Print and shaded views of the part. All mm, measured from the part's lowest x, y and z. A direction names the side the tool comes from. Round coordinates to 2 decimals unless told otherwise and drop trailing zeros. Loops run counter-clockwise (first coordinate to the right, second up) from the corner with the lowest first, then second, coordinate; pieces in that order, holes last. Notation, with made-up numbers: (60, 76.25) -> (84, 76.25) arc R34 cw to (84, 115.25) -> close; hole circle Ø2 at (38.25, 64). An arc over 180 degrees is marked (long way). Use a Markdown table: item, result.
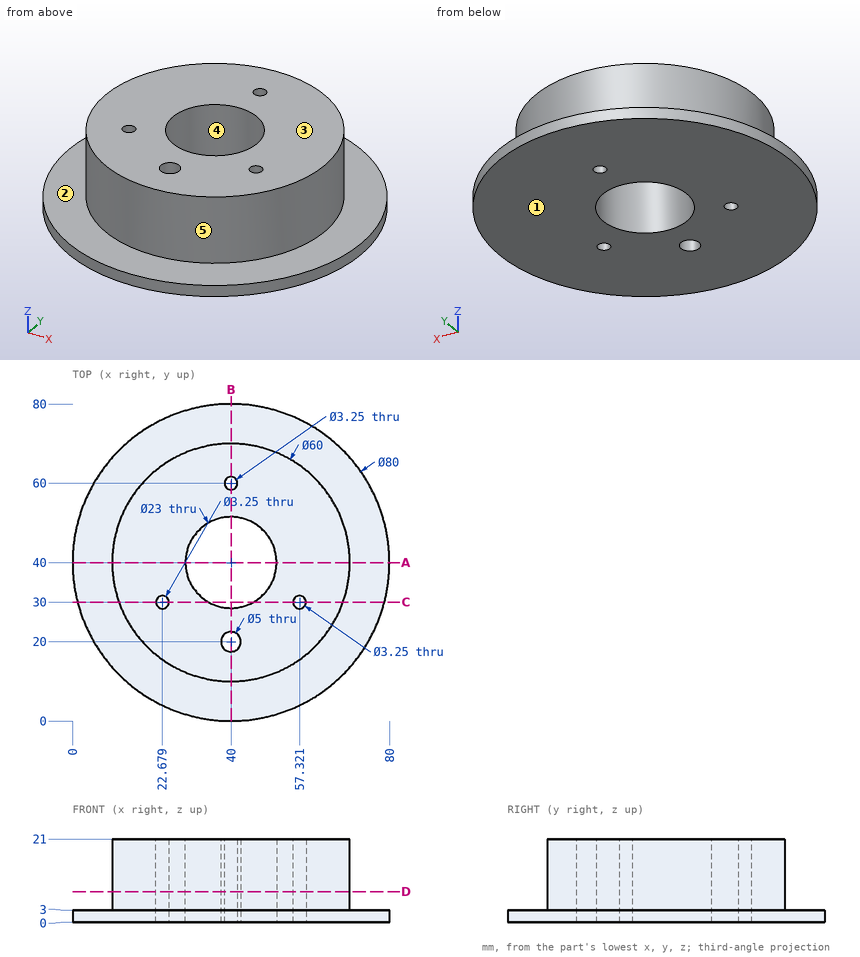
Q1. Tool access for the marked faces 1 and 2: list every direction of +Z, -Z, +X, -X, +Y, -Y with a clear straight run to the whole face (end or side of a thin tool).
Results list:
| item | result |
|---|---|
| face 1 | -Z, +X, -X, +Y, -Y |
| face 2 | +Z |
Q2. Band-saw the part on A-A, the plane y = 40. Give the cut face in (x, z), plus the area to 3 significant figures.
Results list:
| item | result |
|---|---|
| outline | (0, 0) -> (28.5, 0) -> (28.5, 21) -> (10, 21) -> (10, 3) -> (0, 3) -> close; (51.5, 0) -> (80, 0) -> (80, 3) -> (70, 3) -> (70, 21) -> (51.5, 21) -> close |
| area | 837 mm² |
Q3. Drill centre lines: L1, parallel to Y at x = 40, z = 12.25 (1 decimal); L2, parallel to Z at x = 55, y = 6; L3, parallel to X at y = 46, z = 13.75 (1 decimal). Where is each one in solid material? Low to high. Write a range as from..to.
Results list:
| item | result |
|---|---|
| L1 | y = 10..17.5, 22.5..28.5, 51.5..58.4, 61.6..70 |
| L2 | z = 0..3 |
| L3 | x = 10.6..30.2, 49.8..69.4 |
Q4. Flat gauge pins, fed straight in: pin 1 (6 mm diameter, centred on x = 40, y = 20, fed in from +Z); pin 2 (4 mm diameter, centred on x = 17, z = 17.5, fed in from -Y) (1 decimal); pin 3 (6 mm diameter, centred on y = 55.5, z = 4, fed in from -X); pin 4 (2 mm diameter, centred on y = 29.5, z = 3, fed in from +X) (1 decimal). Where does each tip first touch, or does it go through?
Results list:
| item | result |
|---|---|
| pin 1 | stops at z = 21 |
| pin 2 | stops at y = 18.6 |
| pin 3 | stops at x = 2.06 |
| pin 4 | stops at x = 78.9 |
Q5. Band-saw the part on C-C, the plane y = 30. Give the cut face in (x, z) (1 decimal).
Results list:
| item | result |
|---|---|
| outline | (1.3, 0) -> (21.1, 0) -> (21.1, 21) -> (11.7, 21) -> (11.7, 3) -> (1.3, 3) -> close; (24.3, 0) -> (34.3, 0) -> (34.3, 21) -> (24.3, 21) -> close; (45.7, 0) -> (55.7, 0) -> (55.7, 21) -> (45.7, 21) -> close; (58.9, 0) -> (78.7, 0) -> (78.7, 3) -> (68.3, 3) -> (68.3, 21) -> (58.9, 21) -> close |
Q6. Band-saw the part on D-D, the plane z = 7.75. Give the number of separate pieces and of enclosed holes in the cut face, plus the area to 3 significant figures.
Results list:
| item | result |
|---|---|
| separate pieces | 1 |
| enclosed holes | 5 |
| area | 2,370 mm² |
Q7. Band-saw the part on B-B, the plane x = 40. Give the cut face in (y, z) (1 decimal).
Results list:
| item | result |
|---|---|
| outline | (0, 0) -> (17.5, 0) -> (17.5, 21) -> (10, 21) -> (10, 3) -> (0, 3) -> close; (22.5, 0) -> (28.5, 0) -> (28.5, 21) -> (22.5, 21) -> close; (51.5, 0) -> (58.4, 0) -> (58.4, 21) -> (51.5, 21) -> close; (61.6, 0) -> (80, 0) -> (80, 3) -> (70, 3) -> (70, 21) -> (61.6, 21) -> close |
Q8. Pull direction X, two halves, no side cores. Call the marked faces 3, 4 and 5: released by +X, released by -X, zero draft, split by the parting line, or undercut.
Results list:
| item | result |
|---|---|
| face 3 | zero draft |
| face 4 | undercut |
| face 5 | split by the parting line |
